Part print with two shaded views. Sizes in mm from the minimum x, y, z corner. A direction names the side the tool comes from. Round coordinates to 2 decimals unless told otherwise and drop trailing zeros. Write each loop counter-clockwise with the first axis right and the second up, starting at its lowest first coordinate (ties: lowest second). Pieces come first, ordered by that corner, then holes. Notation, with made-up numbers: (8.5, 22.5) - (52.5, 22.5) arc R10 ccw to (52.5, 33.5) - close; hole circle Ø9 at (9, 32.25). An arc over 180 degrees is marked (long way). Answer as a JSON object with one key per item and string values. Group by question number.
Item 1: Which spindle directions (+Z, -Z, +X, -X, +Y, -Y) get a long thin tool onto all of the face, cutting with end or side? Do the marked faces 1, 2 and 3. Say none if no direction does.
Item 2: Two-plate mould, pull along Y, no slides. Class the marked faces 4, 5 and 6: +Y half, -Y half, draft (parallel to the pull), parting line (faces both ways), or undercut.
Item 3: Slice it at D-D, the plane z = 3.75. List the corners of the cut face in (x, y).
Item 4: Slice it at A-A, the plane x = 38. List the corners of the cut face in (y, z).
Item 5: Flat gauge pins, fed straight in: pin 1 (1 mm diameter, centred on y = 8, z = 19, fed in from +X); pin 2 (4 mm diameter, centred on y = 3.5, z = 6.5, fed in from +X); pin 3 (3.5 mm diameter, centred on x = 82, y = 12.5, fed in from +Z). Where does each tip first touch, or does it go through?
Item 6: Probe line 1 (X direction, y = 3.5, z = 4.5); line 2 (X direction, y = 9.5, z = 19.25); line 3 (Z direction, x = 81, y = 6). List the from-to ranges inside material, lowest first. Write a range as from..to.
Item 7: Slice it at C-C, the plane y = 10. List the corners of the cut face in (x, z), then the cut area to 3 significant figures.
Item 8: Slice it at B-B, the plane z = 10. List the corners of the cut face in (x, y).
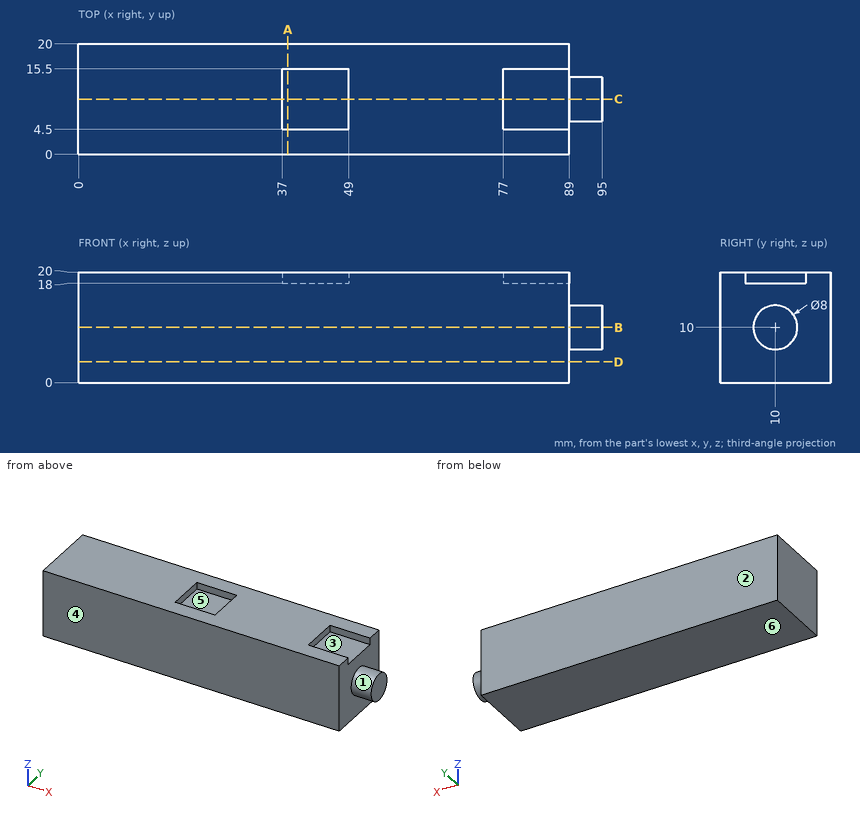
Geometry says:
{
 "1": {"face 1": "+X", "face 2": "+Z, -Z, +X, -X, +Y", "face 3": "+Z, +X"},
 "2": {"face 4": "-Y half", "face 5": "undercut", "face 6": "draft"},
 "3": {"outline": "(0, 0) - (89, 0) - (89, 20) - (0, 20) - close"},
 "4": {"outline": "(0, 0) - (20, 0) - (20, 20) - (15.5, 20) - (15.5, 18) - (4.5, 18) - (4.5, 20) - (0, 20) - close"},
 "5": {"pin 1": "stops at x = 77", "pin 2": "stops at x = 89", "pin 3": "stops at z = 18"},
 "6": {"line 1": "x = 0..89", "line 2": "x = 0..37, 49..77", "line 3": "z = 0..18"},
 "7": {"outline": "(0, 0) - (89, 0) - (89, 6) - (95, 6) - (95, 14) - (89, 14) - (89, 18) - (77, 18) - (77, 20) - (49, 20) - (49, 18) - (37, 18) - (37, 20) - (0, 20) - close", "area": "1,780 mm^2"},
 "8": {"outline": "(0, 0) - (89, 0) - (89, 6) - (95, 6) - (95, 14) - (89, 14) - (89, 20) - (0, 20) - close"}
}
